```python
from build123d import *

# Parameters (mm, degrees)
F0_W     = 25.4
F0_H     = 25.4
F1_DEPTH = 25.4
F2_R     = 4.0005
F3_DEPTH = 25.401
F4_R     = 4.0005
F5_DEPTH = 7.62
F6_R     = 1.905
F7_DEPTH = 25.4


with BuildPart() as f1:
    # F0 (on Front) → F1 (new body)
    with BuildSketch(Plane.XZ):
        with Locations((0, 16.51)):
            Rectangle(F0_W, F0_H)
        Polygon((-25.4, 3.81), (-25.4, 0), (25.4, 0), (25.4, 3.81), (12.7, 3.81), (-12.7, 3.81), align=None)
    extrude(amount=F1_DEPTH)

    # F2 (on face) → F3 (cut, through all)
    with BuildSketch(Plane(origin=(0, 0, 0), x_dir=(-1, 0, 0), z_dir=(0, 1, 0))):
        with Locations((0, 16.51)):
            Circle(F2_R)
    extrude(amount=-F3_DEPTH, mode=Mode.SUBTRACT)

    # F4 (on face) → F5 (cut)
    with BuildSketch(Plane(origin=(0, 0, 0), x_dir=(-1, 0, 0), z_dir=(0, 1, 0))):
        Polygon((7.332348, 16.51), (3.666174, 22.86), (-3.666174, 22.86), (-7.332348, 16.51), (-3.666174, 10.16), (3.666174, 10.16), align=None)
        with Locations((0, 16.51)):
            Circle(F4_R, mode=Mode.SUBTRACT)
    extrude(amount=-F5_DEPTH, mode=Mode.SUBTRACT)

    # F6 (on face) → F7 (cut)
    with BuildSketch(Plane.XY.offset(3.81)):
        with Locations((-19.05, -12.7)):
            Circle(F6_R)
        with Locations((19.05, -12.7)):
            Circle(F6_R)
    extrude(amount=-F7_DEPTH, mode=Mode.SUBTRACT)


solid = f1.part
```
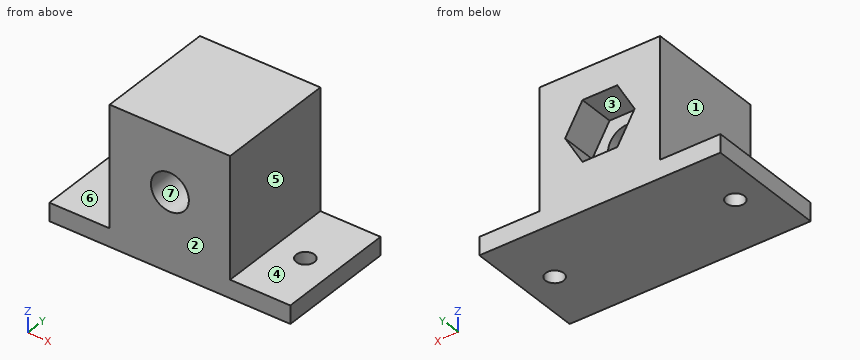
Read the model definition and answer for the solid it produces. Units are mm, in the model's axes. Face numbers are marked on the shaded views. A direction names the side the tool comes from. Coordinates: 2 decimals unless noted, no trailing zeros. Write each loop counter-clockwise with the first axis right and the second up, starting at its lowest first coordinate (ties: lowest second). Pieces come first, ordered by that corner, then holes. Notation, with made-up numbers: (43.25, 8.25) -> (94.25, 8.25) arc R34 cw to (94.25, 39.25) -> close; hole circle Ø3 at (11, 36.5). An arc over 180 degrees is marked (long way). Return JSON: item names as keys, results as strings.
1. A cutting plane is placed at A-A (y = -3.25). Determine the outline of the cut face in (x, z).
Found:
{"outline": "(-25.4, 0) -> (25.4, 0) -> (25.4, 3.81) -> (12.7, 3.81) -> (12.7, 29.21) -> (-12.7, 29.21) -> (-12.7, 3.81) -> (-25.4, 3.81) -> close; hole (-7.33, 16.51) -> (-3.67, 10.16) -> (3.67, 10.16) -> (7.33, 16.51) -> (3.67, 22.86) -> (-3.67, 22.86) -> close"}
2. A tool of negligible diameter and unlimited length cuts with its end or side. For the marked faces 1, 2, 3 and 4, from which of +Z, -Z, +X, -X, +Y, -Y can it reach the whole face along a straight path? Write none if from no direction.
Found:
{"face 1": "+Z, -X, +Y, -Y", "face 2": "+Z, -Z, +X, -X, -Y", "face 3": "+Y", "face 4": "+Z, +X, +Y, -Y"}
3. A cutting plane is placed at C-C (x = 0). Determine the outline of the cut face in (y, z).
Found:
{"outline": "(-25.4, 0) -> (0, 0) -> (0, 10.16) -> (-7.62, 10.16) -> (-7.62, 12.51) -> (-25.4, 12.51) -> close; (-25.4, 20.51) -> (-7.62, 20.51) -> (-7.62, 22.86) -> (0, 22.86) -> (0, 29.21) -> (-25.4, 29.21) -> close"}
4. A cutting plane is placed at D-D (y = -9.25). Determine the outline of the cut face in (x, z), and give its area (3 significant figures).
Found:
{"outline": "(-25.4, 0) -> (25.4, 0) -> (25.4, 3.81) -> (12.7, 3.81) -> (12.7, 29.21) -> (-12.7, 29.21) -> (-12.7, 3.81) -> (-25.4, 3.81) -> close; hole circle Ø8 at (0, 16.51)", "area": "788 mm2"}
5. Each of these flat-tipped pins is pushed along its axis until it touches: P1, Ø1.5, axis at y = -14.5, z = 24, coming from the -X side; P2, Ø12.5, axis at y = -14, z = 13, coming from the +X side; P3, Ø2.5, axis at x = -19.05, y = -12.7, coming from the -Z side; P4, Ø3, axis at x = -14.5, y = -3.5, coming from the +Z side. Where does it stop, or does it pass through?
Found:
{"P1": "x = -12.7", "P2": "x = 12.7", "P3": "through", "P4": "z = 3.81"}
6. Determine the mould class of the marked faces 5, 6 and 7 for opening direction X: pulls with the +X half, pulls with the -X half, needs draft (parallel to the pull), parting line crosses it, or undercut.
Found:
{"face 5": "pulls with the +X half", "face 6": "needs draft", "face 7": "undercut"}
7. Find the intervals of material crossed by line 1 along Z through (x, y) = (0, -20.5); line 2 along Y through (x, z) = (19.05, 3) (3 decimals); line 3 along X through (y, z) = (-13.75, 3), in increasing order. Write a range as from..to.
Found:
{"line 1": "0..12.51, 20.51..29.21", "line 2": "-25.4..-14.605, -10.795..0", "line 3": "-25.4..-20.64, -17.46..17.46, 20.64..25.4"}
8. A cutting plane is placed at B-B (x = -19.05). Determine the outline of the cut face in (y, z) (3 decimals).
Found:
{"outline": "(-25.4, 0) -> (-14.605, 0) -> (-14.605, 3.81) -> (-25.4, 3.81) -> close; (-10.795, 0) -> (0, 0) -> (0, 3.81) -> (-10.795, 3.81) -> close"}
